Build history of the part. All positions in model axes, mm. A direction names the side the tool comes from. Round coordinates to 2 decimals unless told otherwise and drop trailing zeros. Write each question's results on one line, items separated by ' | '.
from build123d import *

# Parameters (mm, degrees)
F1_DEPTH    = 17.78
F2_DEPTH    = 5.08
F3_T1_DEPTH = 35.8062984981
F3_T3_DEPTH = 30.4788212018
F3_T5_DEPTH = 42.8132024584
F3_T7_DEPTH = 47.9220802156


# Not quite as in the source:
# - a fillet or chamfer that OpenCascade refuses, or shapes differently, is made with other operations: its cross-section is extruded or revolved along the edge and cut away or added


with BuildPart() as f1:
    # F0 (on Front) → F1 (new body)
    with BuildSketch(Plane.XZ):
        with BuildLine():
            add(Edge.make_bspline(
                [(-37.0363406837, 14.0804359689), (-35.9072652533, 14.4664877028), (-32.2858897401, 15.7047028462), (-9.9762911381, 14.9349511241), (4.1730021841, 13.4876905203), (11.3340960816, 12.755217962)],
                knots=[0, 0, 0, 0, 0.1828362337, 0.5864255319, 1, 1, 1, 1], degree=3))
            add(Edge.make_bspline(
                [(-40.7805715998, -7.587400265), (-41.1571131004, -3.1737627482), (-41.8654052574, 5.1284956529), (-38.5767054854, 11.224964985), (-37.0363406837, 14.0804359689)],
                knots=[0, 0, 0, 0, 0.5316189046, 1, 1, 1, 1], degree=3))
            add(Edge.make_bspline(
                [(-39.2111837864, -7.587400265), (-39.7343130575, -7.587400265), (-40.2574423287, -7.587400265), (-40.7805715998, -7.587400265)],
                knots=[0, 0, 0, 0, 1.5693878134, 1.5693878134, 1.5693878134, 1.5693878134], degree=3))
            add(Edge.make_bspline(
                [(-39.7181957521, -16.0697158426), (-39.5491917635, -13.2422773167), (-39.380187775, -10.4148387909), (-39.2111837864, -7.587400265)],
                knots=[39.5947721886, 39.5947721886, 39.5947721886, 39.5947721886, 48.0922270247, 48.0922270247, 48.0922270247, 48.0922270247], degree=3))
            Line((-39.7181957521, -16.0697158426), (-34.6953757107, -16.0697158426))
            add(Edge.make_bspline(
                [(18.1377418348, -17.9571639745), (1.0042935619, -17.3535464951), (-17.5619274378, -16.673333322), (-34.6953757107, -16.0697158426)],
                knots=[0, 0, 0, 0, 52.8668210698, 52.8668210698, 52.8668210698, 52.8668210698], degree=3))
            Line((18.1377418348, -17.9571639745), (22.5548642091, -17.9571639745))
            add(Edge.make_bspline(
                [(31.0414787382, 56.6072203219), (29.451074184, 52.0886125693), (26.2723609904, 43.0573519115), (22.6536296154, 29.3346938321), (21.2600863367, 16.9929663306), (21.1386219291, 7.653611923), (21.0411584125, -5.3538743468), (22.1296230711, -14.7801385495), (22.5548642091, -17.9571639745)],
                knots=[0, 0, 0, 0, 0.1361460961, 0.2721127721, 0.3967558164, 0.5055490646, 0.651139282, 0.7233224297, 0.7233224297, 0.7233224297, 0.7233224297], degree=3))
            add(Edge.make_bspline(
                [(22.9297485203, 59.1378286481), (23.9176047114, 59.2712834835), (26.2358281174, 59.584464821), (29.2892185653, 57.692797983), (31.0414787382, 56.6072203219)],
                knots=[0, 0, 0, 0, 0.4261263986, 1, 1, 1, 1], degree=3))
            add(Edge.make_bspline(
                [(11.3340960816, 12.755217962), (11.0324387543, 17.4888695508), (10.3827239426, 27.6842908865), (15.5238608305, 47.2129566198), (20.6106760328, 55.4036857883), (22.9297485203, 59.1378286481)],
                knots=[0, 0, 0, 0, 0.3204519046, 0.6901949001, 1, 1, 1, 1], degree=3))
        make_face()
    extrude(amount=F1_DEPTH)

    # F0 (on Front) → F2 (join)
    with BuildSketch(Plane.XZ):
        with BuildLine():
            Line((-34.6953757107, -16.0697158426), (-39.7181957521, -16.0697158426))
            add(Edge.make_bspline(
                [(-42.0806705952, -55.593945086), (-41.2931789808, -42.4192020049), (-40.5056873665, -29.2444589237), (-39.7181957521, -16.0697158426)],
                knots=[0, 0, 0, 0, 39.5947721886, 39.5947721886, 39.5947721886, 39.5947721886], degree=3))
            add(Edge.make_bspline(
                [(-38.1803736091, -55.593945086), (-39.4804726044, -55.593945086), (-40.7805715998, -55.593945086), (-42.0806705952, -55.593945086)],
                knots=[0, 0, 0, 0, 3.9002969861, 3.9002969861, 3.9002969861, 3.9002969861], degree=3))
            add(Edge.make_bspline(
                [(-34.6953757107, -16.0697158426), (-35.8570416768, -29.2444589237), (-37.018707643, -42.4192020049), (-38.1803736091, -55.593945086)],
                knots=[0, 0, 0, 0, 39.6775743668, 39.6775743668, 39.6775743668, 39.6775743668], degree=3))
        make_face()
        with BuildLine():
            add(Edge.make_bspline(
                [(22.5548642091, -17.9571639745), (23.1406834486, -22.3338868554), (25.110997642, -34.7891360369), (26.7680646459, -47.4091949068), (27.8295651078, -55.4934777319)],
                knots=[0.7233224297, 0.7233224297, 0.7233224297, 0.7233224297, 0.8227631303, 1, 1, 1, 1], degree=3))
            Line((22.5548642091, -17.9571639745), (18.1377418348, -17.9571639745))
            add(Edge.make_bspline(
                [(21.7594448477, -55.4934777319), (21.0663466567, -46.5798409174), (19.8733367549, -31.2370552726), (18.6502547708, -21.8786527932), (18.1377418348, -17.9571639745)],
                knots=[0, 0, 0, 0, 0.5809660006, 1, 1, 1, 1], degree=3))
            add(Edge.make_bspline(
                [(27.8295651078, -55.4934777319), (25.8061916878, -55.4934777319), (23.7828182677, -55.4934777319), (21.7594448477, -55.4934777319)],
                knots=[0, 0, 0, 0, 6.0701202601, 6.0701202601, 6.0701202601, 6.0701202601], degree=3))
        make_face()
    extrude(amount=F2_DEPTH)

    # F3: fillet of radius 5.08 on 4 edges, made by hand

    # F3_s2 → F3_t1 (cut)
    with BuildSketch(Plane.XZ.offset(-9.0131492491)):
        with BuildLine():
            ThreePointArc((-41.0654329019, -3.9934120152), (-40.5113634996, -5.9828767727), (-39.2111837864, -7.587400265))
            Line((-39.2111837864, -7.587400265), (-39.2754713457, -7.666074719))
            ThreePointArc((-39.2754713457, -7.666074719), (-39.9958776931, -7.689000265), (-40.7805715998, -7.689000265))
            Line((-40.7805715998, -7.689000265), (-40.8818038663, -7.5960367127))
            ThreePointArc((-40.8818038663, -7.5960367127), (-41.0323979759, -5.7992458414), (-41.1668054436, -4.0002067042))
            Line((-41.1668054436, -4.0002067042), (-41.0654329019, -3.9934120152))
        make_face()
    extrude(amount=F3_T1_DEPTH, mode=Mode.SUBTRACT)

    # F3_s4 → F3_t3 (cut)
    with BuildSketch(Plane.XZ.offset(-6.3494106009)):
        with BuildLine():
            ThreePointArc((-34.5963046101, 14.7851531861), (-36.6248709598, 13.860065118), (-38.061951969, 12.1554632461))
            Line((-38.061951969, 12.1554632461), (-38.1521078254, 12.2023085399))
            ThreePointArc((-38.1521078254, 12.2023085399), (-37.6424780921, 13.1678308874), (-37.1257598745, 14.1286725558))
            Line((-37.1257598745, 14.1286725558), (-37.0692112747, 14.1765717284))
            ThreePointArc((-37.0692112747, 14.1765717284), (-35.8572472499, 14.5711412658), (-34.6171475194, 14.8845922787))
            Line((-34.6171475194, 14.8845922787), (-34.5963046101, 14.7851531861))
        make_face()
    extrude(amount=F3_T3_DEPTH, mode=Mode.SUBTRACT)

    # F3_s6 → F3_t5 (cut)
    with BuildSketch(Plane.XZ.offset(-12.5166012292)):
        with BuildLine():
            ThreePointArc((27.8862106757, 58.4307700125), (24.2228232961, 58.7447859797), (21.3071174751, 56.5047697552))
            Line((21.3071174751, 56.5047697552), (21.220258421, 56.5574771049))
            ThreePointArc((21.220258421, 56.5574771049), (22.0285709469, 57.8767827762), (22.8434388423, 59.1914308821))
            Line((22.8434388423, 59.1914308821), (22.9161463902, 59.2385140098))
            ThreePointArc((22.9161463902, 59.2385140098), (25.4817069799, 59.3415947788), (27.9309334856, 58.5219973674))
            Line((27.9309334856, 58.5219973674), (27.8862106757, 58.4307700125))
        make_face()
    extrude(amount=F3_T5_DEPTH, mode=Mode.SUBTRACT)

    # F3_s8 → F3_t7 (cut)
    with BuildSketch(Plane.XZ.offset(-15.0710401078)):
        with BuildLine():
            ThreePointArc((29.6134478053, 52.5339448765), (29.1735899714, 56.8129265835), (25.6089175294, 59.2204709225))
            Line((25.6089175294, 59.2204709225), (25.6247878066, 59.3208237715))
            ThreePointArc((25.6247878066, 59.3208237715), (28.4954140197, 58.2321967662), (31.0949864807, 56.6935886118))
            Line((31.0949864807, 56.6935886118), (31.1373157967, 56.5734887606))
            ThreePointArc((31.1373157967, 56.5734887606), (30.4214522449, 54.5375989985), (29.709408688, 52.5005672046))
            Line((29.709408688, 52.5005672046), (29.6134478053, 52.5339448765))
        make_face()
    extrude(amount=F3_T7_DEPTH, mode=Mode.SUBTRACT)

    # F5: F1 across plane


with BuildPart() as f1_1:
    add(f1.part)
    add(f1.part.mirror(Plane(origin=(-3.442122023, -17.78, 6.1004007624), x_dir=(1, 0, 0), z_dir=(0, -1, 0))))


solid = f1_1.part
(1) Drill centre lines: probe 1 along Y at (x, z) = (-36.5, -35.5); probe 2 along X at (y, z) = (-29, 7); probe 3 along Z at (x, y) = (-12, -5). Where is each one in solid material? Low to high. Write a range as [from, to].
Worked answers:
probe 1: y = [-35.56, -30.48], [-5.08, 0] | probe 2: x = [-40.28, 21.14] | probe 3: z = [-16.88, 14.79]
(2) Tool access for faces 5 (the flat face through (23, -30.48, -36)), 6 (the cylindrical face through (23.871, -18.029, 58.628)), 7 (the flat face through (-37, -18, -16.07)): list every direction of +Z, -Z, +X, -X, +Y, -Y with a clear straight run to the whole face (end or side of a thin tool).
Worked answers:
face 5: -Z, +X, -X | face 6: +Z, +Y, -Y | face 7: -Z, -X
(3) Two-plate mould, pull along Z, no slides. Class faces 1 (the flat face through (-39.47, -18.03, -11.89)), 2 (the cylindrical face through (-40.525, -18.029, -5.957)), 3 (the flat face through (20, -18, -17.957)), 4 (the flat face through (-38, -30.48, -36)): released by +Z, released by -Z, zero draft, split by the parting line, or undercut.
Worked answers:
face 1: undercut | face 2: undercut | face 3: released by -Z | face 4: zero draft
(4) Slice it at A-A, the plane z = -46.5. State how many separate pieces and enclosed holes the cut face has, and give its area (3 significant figures).
Worked answers:
separate pieces: 4 | enclosed holes: 0 | area: 99.0 mm2
(5) Flat gauge pins, fed straight in: pin 1 Ø1 at (x, y) = (-23.5, -22) entering from +Z; pin 2 Ø3.5 at (x, y) = (21, -19.5) entering from -Z; pin 3 Ø2.5 at (x, y) = (-36.5, -19) entering from -Z. Where does each tip first touch, or does it go through?
Worked answers:
pin 1: stops at z = 15.3 | pin 2: stops at z = -17.96 | pin 3: stops at z = -16.07
